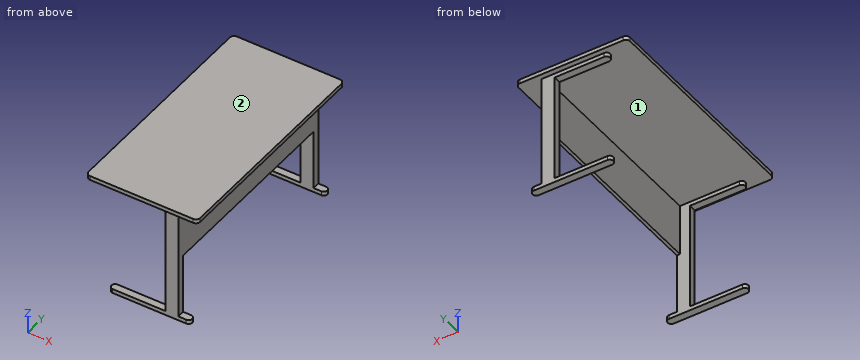
```python
from build123d import *

# Parameters (mm, degrees)
F1_DEPTH = 25.4
F3_DEPTH = 25.4
F5_DEPTH = 288.925
F6_W     = 79.375
F6_H     = 44.45
F7_DEPTH = 368.3
F9_DEPTH = 25.4


with BuildPart() as f1:
    # F0 (on Top) → F1 (new body)
    with BuildSketch(Plane.XY):
        with BuildLine():
            ThreePointArc((339.725, 650.875), (332.285512, 668.835512), (314.325, 676.275))
            Line((314.325, 676.275), (-314.325, 676.275))
            ThreePointArc((-314.325, 676.275), (-332.285512, 668.835512), (-339.725, 650.875))
            Line((-339.725, 650.875), (-339.725, -650.875))
            ThreePointArc((-339.725, -650.875), (-332.285512, -668.835512), (-314.325, -676.275))
            Line((-314.325, -676.275), (314.325, -676.275))
            ThreePointArc((314.325, -676.275), (332.285512, -668.835512), (339.725, -650.875))
            Line((339.725, -650.875), (339.725, 650.875))
        make_face()
    extrude(amount=F1_DEPTH)

    # F2 (on face) → F3 (join)
    with BuildSketch(Plane(origin=(0, 0, 0), x_dir=(1, 0, 0), z_dir=(0, 0, -1))):
        with BuildLine():
            ThreePointArc((-177.8, 644.525), (-200.025, 622.3), (-177.8, 600.075))
            Line((-177.8, 600.075), (184.15, 600.075))
            Line((184.15, 600.075), (184.15, -600.075))
            Line((184.15, -600.075), (-177.8, -600.075))
            ThreePointArc((-177.8, -600.075), (-200.025, -622.3), (-177.8, -644.525))
            Line((-177.8, -644.525), (203.2, -644.525))
            Line((203.2, -644.525), (203.2, 644.525))
            Line((203.2, 644.525), (-177.8, 644.525))
        make_face()
    extrude(amount=F3_DEPTH)

    # F4 (on face) → F5 (join)
    with BuildSketch(Plane(origin=(0, 0, -25.4), x_dir=(1, 0, 0), z_dir=(0, 0, -1))):
        Polygon((123.825, 644.525), (123.825, 600.075), (184.15, 600.075), (184.15, -600.075), (123.825, -600.075), (123.825, -644.525), (203.2, -644.525), (203.2, 644.525), align=None)
    extrude(amount=F5_DEPTH)

    # F6 (on face) → F7 (join)
    with BuildSketch(Plane(origin=(0, 0, -314.325), x_dir=(1, 0, 0), z_dir=(0, 0, -1))):
        with Locations((163.5125, -622.3)):
            Rectangle(F6_W, F6_H)
        with Locations((163.5125, 622.3)):
            Rectangle(F6_W, F6_H)
    extrude(amount=F7_DEPTH)

    # F8 (on face) → F9 (join)
    with BuildSketch(Plane(origin=(0, 0, -682.625), x_dir=(1, 0, 0), z_dir=(0, 0, -1))):
        with BuildLine():
            ThreePointArc((250.825, 600.075), (273.05, 622.3), (250.825, 644.525))
            Line((250.825, 644.525), (-196.85, 644.525))
            ThreePointArc((-196.85, 644.525), (-219.075, 622.3), (-196.85, 600.075))
            Line((-196.85, 600.075), (250.825, 600.075))
        make_face()
        with BuildLine():
            Line((250.825, -600.075), (-196.85, -600.075))
            ThreePointArc((-196.85, -600.075), (-219.075, -622.3), (-196.85, -644.525))
            Line((-196.85, -644.525), (250.825, -644.525))
            ThreePointArc((250.825, -644.525), (273.05, -622.3), (250.825, -600.075))
        make_face()
    extrude(amount=F9_DEPTH)


solid = f1.part
```
Check sheet for the modelled part. Datum: model origin and axes. Units: mm. Face numbers are marked on the shaded views. Coordinates: 2 decimals unless noted, no trailing zeros. Loops run counter-clockwise (first coordinate to the right, second up) from the corner with the lowest first, then second, coordinate; pieces in that order, holes last.
1) Sectioned sample at C-C (y = -622.3). Record the boundary of the cut face in (x, z) (3 decimals).
2) Sectioned sample at D-D (z = -235.5). Record the boundary of the cut face in (x, y) (3 decimals), and give its area (3 significant figures).
3) Sectioned sample at A-A (z = -525). Record the boundary of the cut face in (x, y) (3 decimals), and give its area (3 significant figures).
4) Release check for a two-part mould opening along Y. For the marked faces 1 and 2 record: released by +Y, released by -Y, zero draft, split by the parting line, or undercut.
5) Material ranges on probe 1 along Y at (x, z) = (25.5, -22.5) (3 decimals); probe 2 along Z at (x, y) = (134, 159); probe 3 along X at (y, z) = (408.5, -180.5), recorded low to high.
6) Gauge pin test, flat ends, axial feed: pin 1 (12 mm diameter, centred on y = -37, z = -282.5, fed in from +X); pin 2 (21 mm diameter, centred on x = 197.5, y = -288.5, fed in from -Z) (3 decimals); pin 3 (2 mm diameter, centred on y = 350.5, z = -141, fed in from -X). Record the tip position at first contact, or that the pin passes through.
7) Sectioned sample at B-B (x = 60.5). Record the boundary of the cut face in (y, z) (3 decimals), and give its area (3 significant figures).
Check sheet entries:
1. outline: (-339.725, 0) - (-200.025, 0) - (-200.025, -25.4) - (123.825, -25.4) - (123.825, -682.625) - (-219.075, -682.625) - (-219.075, -708.025) - (273.05, -708.025) - (273.05, -682.625) - (203.2, -682.625) - (203.2, 0) - (339.725, 0) - (339.725, 25.4) - (-339.725, 25.4) - close
2. outline: (123.825, -644.525) - (203.2, -644.525) - (203.2, 644.525) - (123.825, 644.525) - (123.825, 600.075) - (184.15, 600.075) - (184.15, -600.075) - (123.825, -600.075) - close
2. area: 29,900 mm2
3. outline: (123.825, -644.525) - (203.2, -644.525) - (203.2, -600.075) - (123.825, -600.075) - close; (123.825, 600.075) - (203.2, 600.075) - (203.2, 644.525) - (123.825, 644.525) - close
3. area: 7,060 mm2
4. face 1: undercut
4. face 2: zero draft
5. probe 1: y = -644.525 to -600.075, 600.075 to 644.525
5. probe 2: z = 0 to 25.4
5. probe 3: x = 184.15 to 203.2
6. pin 1: stops at x = 203.2
6. pin 2: stops at z = -314.325
6. pin 3: stops at x = 184.15
7. outline: (-676.275, 0) - (-644.525, 0) - (-644.525, -25.4) - (-600.075, -25.4) - (-600.075, 0) - (600.075, 0) - (600.075, -25.4) - (644.525, -25.4) - (644.525, 0) - (676.275, 0) - (676.275, 25.4) - (-676.275, 25.4) - close; (-644.525, -708.025) - (-600.075, -708.025) - (-600.075, -682.625) - (-644.525, -682.625) - close; (600.075, -708.025) - (644.525, -708.025) - (644.525, -682.625) - (600.075, -682.625) - close
7. area: 38,900 mm2
